Part model, mm, in its own coordinate system. Face numbers are marked on the shaded views. A direction names the side the tool comes from. Coordinates: 2 decimals unless noted, no trailing zeros. Order: outer loops, then holes, each group sorted by start corner. A loop starts at its lowest first (then second) coordinate and runs counter-clockwise, first axis right, second up. Notation, with made-up numbers: (7, -24) - (53, -24) arc R33 ccw to (53, 9) - close; hole circle Ø4 at (0.25, 1.5). An arc over 180 degrees is marked (long way). Use a Markdown table: item, result. Add a question column.
1) Wall check: L1, parallel to Z at x = -55.5, y = 13.5; L2, parallel to X at y = 5.75, z = -32; L3, parallel to Y at x = -40, z = -49.5. Give the ranges that are in metal, low to high. Write a range as [from, to].
2) Two-plate mould, pull along X, no slides. Class the marked faces 3, 4 and 5: +X half, -X half, draft (parallel to the pull), parting line (faces both ways), or undercut.
3) Drop a flat-ended pin along its axis: P1, Ø16.5, axis at x = -49.5, z = -31.5, coming from the +Y side. Give the stop position or say it passes through.
4) Saw through at A-A on y = 3.5. List the corners of the cut face in (x, z), then the cut area to 3 significant figures.
5) Saw through at B-B on x = -44.5. List the corners of the cut face in (y, z), then the cut area to 3 significant figures.
6) Tool access for the marked faces 1 and 2: list every direction of +Z, -Z, +X, -X, +Y, -Y with a clear straight run to the whole face (end or side of a thin tool).
7) Saw through at C-C on z = -19. List the corners of the cut face in (x, y).
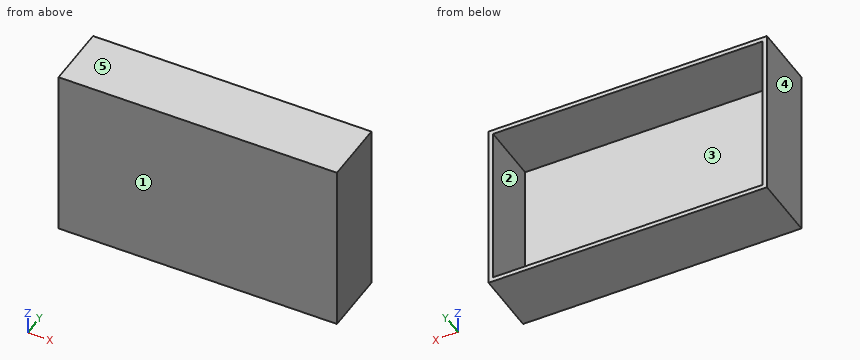
```python
from build123d import *

# Parameters (mm, degrees)
ESBO_O1_W                = 90
ESBO_O1_H                = 55
RESSALTO_EXTRUS_O1_DEPTH = 20
CASCA1_T                 = 1.5


with BuildPart() as part:
    # Esboço1 → Ressalto-extrusão1 (new body)
    with BuildSketch(Plane(origin=(0, 0, 0), x_dir=(1, 0, 0), z_dir=(0, 1, 0))):
        with Locations((-44.890471739, 35.305061179)):
            Rectangle(ESBO_O1_W, ESBO_O1_H)
    extrude(amount=RESSALTO_EXTRUS_O1_DEPTH)

    # Casca1
    casca1_openings = [part.faces().sort_by_distance(p)[0] for p in [
        (-44.890471739, 20, -35.305061179),
    ]]
    offset(amount=CASCA1_T, openings=casca1_openings, kind=Kind.INTERSECTION)


solid = part.part
```
Results are:
| question | item | result |
|---|---|---|
| 1 | L1 | [-64.31, -62.81], [-7.81, -6.31] |
| 1 | L2 | [-91.39, -89.89], [0.11, 1.61] |
| 1 | L3 | [-1.5, 0] |
| 2 | face 3 | undercut |
| 2 | face 4 | -X half |
| 2 | face 5 | draft |
| 3 | P1 | y = 0 |
| 4 | outline | (-91.39, -64.31) - (1.61, -64.31) - (1.61, -6.31) - (-91.39, -6.31) - close; hole (-89.89, -62.81) - (0.11, -62.81) - (0.11, -7.81) - (-89.89, -7.81) - close |
| 4 | area | 444 mm2 |
| 5 | outline | (-1.5, -64.31) - (20, -64.31) - (20, -62.81) - (0, -62.81) - (0, -7.81) - (20, -7.81) - (20, -6.31) - (-1.5, -6.31) - close |
| 5 | area | 147 mm2 |
| 6 | face 1 | +Z, -Z, +X, -X, -Y |
| 6 | face 2 | +Y |
| 7 | outline | (-91.39, -1.5) - (1.61, -1.5) - (1.61, 20) - (0.11, 20) - (0.11, 0) - (-89.89, 0) - (-89.89, 20) - (-91.39, 20) - close |
